For this review, take the finished solid that the model builds, in its own axes (mm). Give positions to 0.01 mm unless a question says otherwise; leave off trailing zeros. Loops run counter-clockwise (first coordinate to the right, second up) from the corner with the lowest first, then second, coordinate; pieces in that order, holes last.
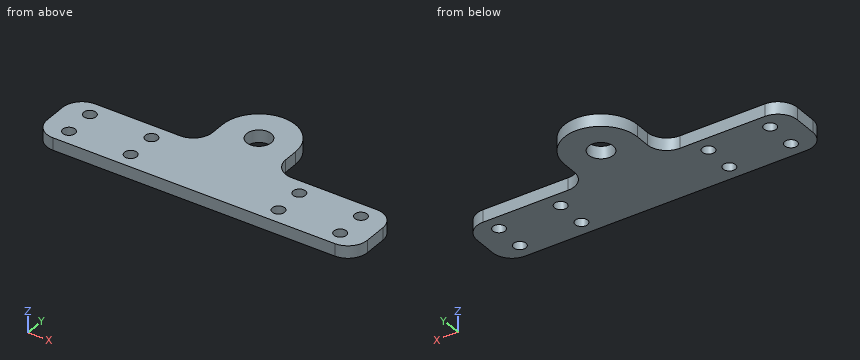
```python
from build123d import *

# Parameters (mm, degrees)
SKETCH1_R           = 3.175
SKETCH1_R_2         = 1.5875
BOSS_EXTRUDE1_DEPTH = 3.175
FILLET1_R           = 5


with BuildPart() as part:
    # Sketch1 → Boss-Extrude1 (new body)
    with BuildSketch(Plane.XY):
        with BuildLine():
            Line((-41.275, -8.7), (-14.398, -8.7))
            ThreePointArc((-14.398, -8.7), (-10.862466094, -7.235533906), (-9.398, -3.7))
            Line((-9.398, -3.7), (-9.398, 0))
            ThreePointArc((-9.398, 0), (0, 9.398), (9.398, 0))
            Line((9.398, 0), (9.398, -3.7))
            ThreePointArc((9.398, -3.7), (10.862466094, -7.235533906), (14.398, -8.7))
            Line((14.398, -8.7), (41.275, -8.7))
            Line((41.275, -8.7), (41.275, -24.575))
            Line((41.275, -24.575), (-41.275, -24.575))
            Line((-41.275, -24.575), (-41.275, -8.7))
        make_face()
        Circle(SKETCH1_R, mode=Mode.SUBTRACT)
        with Locations((-34.925, -12.7)):
            Circle(SKETCH1_R_2, mode=Mode.SUBTRACT)
        with Locations((-34.925, -20.575)):
            Circle(SKETCH1_R_2, mode=Mode.SUBTRACT)
        with Locations((-19.05, -12.7)):
            Circle(SKETCH1_R_2, mode=Mode.SUBTRACT)
        with Locations((-19.05, -20.575)):
            Circle(SKETCH1_R_2, mode=Mode.SUBTRACT)
        with Locations((19.05, -20.575)):
            Circle(SKETCH1_R_2, mode=Mode.SUBTRACT)
        with Locations((19.05, -12.7)):
            Circle(SKETCH1_R_2, mode=Mode.SUBTRACT)
        with Locations((34.925, -20.575)):
            Circle(SKETCH1_R_2, mode=Mode.SUBTRACT)
        with Locations((34.925, -12.7)):
            Circle(SKETCH1_R_2, mode=Mode.SUBTRACT)
    extrude(amount=BOSS_EXTRUDE1_DEPTH)

    # Fillet1
    fillet1_edges = [part.edges().sort_by_distance(p)[0] for p in [
        (-41.275, -8.7, 1.5875),
        (41.275, -8.7, 1.5875),
        (41.275, -24.575, 1.5875),
        (-41.275, -24.575, 1.5875),
    ]]
    fillet(fillet1_edges, radius=FILLET1_R)


solid = part.part
```
Item 1: Take a section at C-C on z = 2.3. State how many separate pieces and enclosed holes the cut face has, and give its area (3 significant figures).
Answer:
separate pieces: 1
enclosed holes: 9
area: 1,510 mm2
Item 2: Clearance check with flat-ended pins moving along their axes: pin 1 Ø1.5 at (x, z) = (-30.5, 2.5) entering from +Y; pin 2 Ø1 at (y, z) = (-1.5, 1) entering from -X; pin 3 Ø1.5 at (y, z) = (-3.5, 2) entering from +X. State where each tip first meets the part, or that it passes through.
Answer:
pin 1: stops at y = -8.7
pin 2: stops at x = -9.4
pin 3: stops at x = 9.43
Item 3: For L1, parallel to Y at x = -19.05, z = 0.8 (1 decimal); L2, parallel to Y at x = -19.5, z = 2.55 (3 decimals); L3, parallel to X at y = -11.5, z = 2.95, list the stretches that pass through material, from the lowest coordinate up.
Answer:
L1: y = -24.6 to -22.2, -19 to -14.3, -11.1 to -8.7
L2: y = -24.575 to -22.097, -19.053 to -14.222, -11.178 to -8.7
L3: x = -40.76 to -35.96, -33.89 to -20.09, -18.01 to 18.01, 20.09 to 33.89, 35.96 to 40.76
Item 4: Take a section at B-B on x = 0. Give the boundary of the cut face in (y, z) (3 decimals).
Answer:
outline: (-24.575, 0) - (-3.175, 0) - (-3.175, 3.175) - (-24.575, 3.175) - close; (3.175, 0) - (9.398, 0) - (9.398, 3.175) - (3.175, 3.175) - close
Item 5: Take a section at D-D on y = -12.7. Give the boundary of the cut face in (x, z) (1 decimal).
Answer:
outline: (-41.2, 0) - (-36.5, 0) - (-36.5, 3.2) - (-41.2, 3.2) - close; (-33.3, 0) - (-20.6, 0) - (-20.6, 3.2) - (-33.3, 3.2) - close; (-17.5, 0) - (17.5, 0) - (17.5, 3.2) - (-17.5, 3.2) - close; (20.6, 0) - (33.3, 0) - (33.3, 3.2) - (20.6, 3.2) - close; (36.5, 0) - (41.2, 0) - (41.2, 3.2) - (36.5, 3.2) - close
Item 6: Take a section at A-A on x = -19.05. Give the boundary of the cut face in (y, z) (1 decimal).
Answer:
outline: (-24.6, 0) - (-22.2, 0) - (-22.2, 3.2) - (-24.6, 3.2) - close; (-19, 0) - (-14.3, 0) - (-14.3, 3.2) - (-19, 3.2) - close; (-11.1, 0) - (-8.7, 0) - (-8.7, 3.2) - (-11.1, 3.2) - close
